Geometry: final body of the model. Coordinates: model frame, mm. Face numbers are marked on the shaded views. A direction names the side the tool comes from. Coordinates: 2 decimals unless noted, no trailing zeros. Order: outer loops, then holes, each group sorted by start corner. A loop starts at its lowest first (then second) coordinate and runs counter-clockwise, first axis right, second up. Notation, with made-up numbers: (-17.75, 15.25) - (-5.75, 15.25) arc R6 ccw to (-5.75, 19.25) - close; hole circle Ø10 at (65, -2.75). An arc over 180 degrees is marked (long way). Use a Markdown table: item, result. Add a question column.
Autodesk Inventor part; units mm, degrees
ref_plane "Work Plane1" through (30, 0, 0) normal (0, -0.5, 0.866) x (1, 0, 0)
ref_plane "YZ Plane" through (0, 0, 0) normal (1, 0, 0) x (0, 1, 0)
ref_plane "XZ Plane" through (0, 0, 0) normal (0, 1, 0) x (-1, 0, 0)
sketch "Sketch1" plane through (0, 0, 0) normal (0, 0, 1) x (1, 0, 0)
  line L0 (-0.0667, 0) -> (10, 0)
  line L1 (10, 0) -> (10, 2)
  line L2 (10, 2) -> (1.4, 2)
  line L3 (1.4, 2) -> (0.9706, 2)
  line L4 (0.9706, 2) -> (0, 2)
  line L5 (0, 2) -> (0, 3.8)
  line L6 (0, 3.8) -> (-2.2, 3.8)
  line L7 (-2.2, 3.8) -> (-2.2, 1.4434)
  line L8 (-2.2, 1.4434) -> (-0.9, 1.4434)
  line L9 (-0.9, 1.4434) -> (-0.0667, 0)
  line L10 (-4.64, 0) -> (12.44, 0)
  line L11 (0, -0.76) -> (0, 4.56)
  line L12 (1.4, 2) -> (0, 2) construction
  dimension "d0" = 8.6
  dimension "d1" = 0.4294
  dimension "d2" = 2.2
  dimension "d3" = 1.3
  dimension "d4" = 60
  dimension "d5" = 4
  dimension "d6" = 4
  dimension "d7" = 2.8868
  dimension "d8" = 7.6
  dimension "d19" = 10
revolve "Body" add sketch "Sketch1" angle 360 about axis through (-0.0667, 0, 0) along (1, 0, 0)
sketch "Sketch2" plane through (-2.2, 0, 0) normal (-1, 0, 0) x (0, 0, 1)
  circle A0 centre (0, 0) radius 1.4434
  line L0 (0, -5.32) -> (0, 5.32)
  line L1 (-5.32, 0) -> (5.32, 0)
  line L2 (1.4434, 0) -> (0.7217, -1.25)
  line L3 (0.7217, -1.25) -> (-0.7217, -1.25)
  line L4 (-0.7217, -1.25) -> (-1.4434, 0)
  line L5 (-1.4434, 0) -> (-0.7217, 1.25)
  line L6 (-0.7217, 1.25) -> (0.7217, 1.25)
  line L7 (0.7217, 1.25) -> (1.4434, 0)
extrude "Slot" add sketch "Sketch2" against normal up to next contours L7 A0 | A0 L2 | L6 L0 A0 | A0 L0 L3 | L0 L6 A0 | A0 L3 L0 | L4 A0 | A0 L5
fillet "Fillet1" radius 1.82 1 edges at (-2.2, -3.8, 0)
thread "Thread"
chamfer "Chamfer1" distance 0.4294 distance2 0.4294 1 edges at (10, -2, 0) measured on face at (10, 0.556, 0.0273)
fillet "Fillet2" radius 0.2 1 edges at (0, -2, 0)
ref_plane "Work Plane1" through (30, 0, 0) normal (0, -0.5, 0.866) x (1, 0, 0)
equation "\"d0\" = GEL"
equation "\"d1\" = GAL"
equation "\"d2\" = KOH"
equation "\"d3\" = INTI"
equation "\"d5\" = GD"
equation "\"d6\" = BDM"
equation "\"d7\" = 1.1547 * SW"
equation "\"d8\" = KOD"
equation "\"d19\" = NLG"
equation "\"d16\" = RR"
equation "\"d12\" = GEL"
equation "\"d14\" = -0.5 * SPD + 0.5 * GD"
equation "\"d15\" = GUL"
equation "\"d29\" = R"
equation "\"GD\" = NND"
equation "\"NLG\" = 10"
equation "\"GEL\" = 8.6"
equation "\"KOD\" = 7.6"
equation "\"KOH\" = 2.2"
equation "\"INTI\" = 1.3"
equation "\"GAL\" = 0.61345 * PTC"
equation "\"GUL\" = 0.61345 * PTC"
equation "\"BDM\" = NND"
equation "\"SW\" = 2.5"
equation "\"RR\" = 1.82"
equation "\"SPD\" = 3.14117"
equation "\"d28\" = R"
equation "\"R\" = 0.2"
equation "\"TOA\" = 30deg"
equation "\"THREADDIA\" = 4"
equation "\"KOD1\" = KOD - 2 * RR"
equation "\"PTC\" = 0.7"
equation "\"NND\" = 4"
equation "\"E0\" = 1.155 * SW"
equation "\"GD1\" = THREADDIA - 1.2269 * PTC"
properties part number "ANSI B18.3.4M - M4 x 0.7 x 10, FHSBHCSM" material "Steel, Mild"
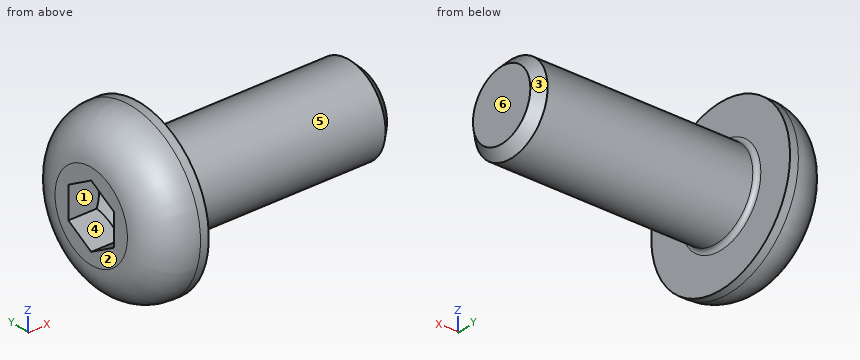
1) Set-up query: the marked faces 4, 5 and 6. Return all of +Z, -Z, +X, -X, +Y, -Y with unobstructed straight access to the full face (end or side cutting, diameter ignored); none if empty.
2) Pin query (flat end, axial travel): pin 1 (2 mm diameter, centred on x = 8, y = -2, fed in from +Z); pin 2 (2 mm diameter, centred on x = -0.5, y = -1.5, fed in from -Z); pin 3 (2 mm diameter, centred on x = 5.5, y = -1.5, fed in from -Z). Return the tip coordinate at first contact, or that it passes through.
3) Section A-A (x = 1.5). Return loops of the section in (y, z).
4) Draft query along Z for the marked faces 1, 2 and 3. Return one class per face: pulls with the +Z half, pulls with the -Z half, needs draft (parallel to the pull), parting line crosses it, or undercut.
5) Ray query, line 1 along Z through (x, y) = (3.75, 0); line 2 along X through (y, z) = (0.5, -0.5); line 3 along Z through (x, y) = (-1.5, 0.75). Return the intervals inside material, ascending.
Values follow:
| question | item | result |
|---|---|---|
| 1 | face 4 | -X |
| 1 | face 5 | +X |
| 1 | face 6 | +Z, -Z, +X, +Y, -Y |
| 2 | pin 1 | stops at z = 1.73 |
| 2 | pin 2 | stops at z = -3.77 |
| 2 | pin 3 | stops at z = -1.94 |
| 3 | outline | circle Ø4 at (0, 0) |
| 4 | face 1 | undercut |
| 4 | face 2 | needs draft |
| 4 | face 3 | parting line crosses it |
| 5 | line 1 | z = -2 to 2 |
| 5 | line 2 | x = -0.47 to 10 |
| 5 | line 3 | z = -3.33 to -1.01, 1.01 to 3.33 |
